The model under review builds one solid part; all positions refer to its coordinate system, in mm. A direction names the side the tool comes from. Give positions to 0.01 mm unless a question says otherwise; leave off trailing zeros. Write each loop counter-clockwise with the first axis right and the second up, starting at its lowest first coordinate (ties: lowest second). Pieces come first, ordered by that corner, then holes.
Autodesk Inventor part; units mm, degrees
ref_plane "YZ Plane" through (0, 0, 0) normal (1, 0, 0) x (0, 1, 0)
ref_plane "XZ Plane" through (0, 0, 0) normal (0, 1, 0) x (-1, 0, 0)
ref_plane "XY Plane" through (0, 0, 0) normal (0, 0, 1) x (1, 0, 0)
ref_plane "Work Plane1" through (0, 0, 0) normal (0, 0, 1) x (1, 0, 0)
sketch "Sketch1" plane through (0, 0, 0) normal (0, 0, 1) x (1, 0, 0)
  line L0 (8.0002, 76.1) -> (3.2502, 76.1) construction
  line L1 (3.2502, 90.8) -> (3.2502, 103.5) construction
  line L2 (-17.75, 107.5) -> (-17.75, -107.5) construction
  line L3 (17.75, 107.5) -> (-17.75, 107.5) construction
  line L4 (1.9802, 107.5) -> (-17.75, 107.5)
  line L5 (-17.75, 107.5) -> (-17.75, 74.83)
  line L6 (-17.75, 74.83) -> (1.9802, 74.83)
  line L7 (1.9802, 74.83) -> (1.9802, 107.5)
  line L8 (-17.75, 74.83) -> (17.75, 74.83)
  line L9 (17.75, 74.83) -> (17.75, -52.17)
  line L10 (17.75, -52.17) -> (-17.75, -52.17)
  line L11 (-17.75, -52.17) -> (-17.75, 74.83)
  point P0 (0, 0)
  dimension "d1" = 1.27
  dimension "d2" = 1.27
  dimension "d5" = 127
extrude "Extrusion1" add sketch "Sketch1" along normal blind 2.54
sketch "Sketch2" plane through (0, 0, 2.54) normal (0, 0, 1) x (1, 0, 0)
  circle A0 centre (9.0001, 13.4819) radius 34.925 construction
  line L0 (12.3751, 101.9) -> (12.3751, 92.4) construction
  line L1 (5.6252, 92.4) -> (5.6252, 101.9) construction
  line L2 (-23.5916, 26.0332) -> (5.6252, 101.9) construction
  line L3 (41.5918, 26.0331) -> (12.3751, 101.9) construction
  point P0 (0, 0)
sketch "Sketch3" plane through (0, 0, 2.54) normal (0, 0, 1) x (1, 0, 0)
  circle A0 centre (9.0001, 13.4819) radius 44.45 construction
  point P0 (0, 0)
properties part number "horizontal spool mount bottom"
1) Consider section A-A, the plane z = 2. Give the boundary of the cut face in (x, y), then the cut area to 3 significant figures.
2) Insertion check: pin 1 (0.8 mm diameter, centred on x = 11.5, z = 1, fed in from +Y); pin 2 (1.3 mm diameter, centred on y = 91, z = 1, fed in from +X). Each pin has a flat end and moves straight along its axis. Give the tip position at first contact, or say it passes through.
3) Consider section B-B, the plane x = 13.5. Give the boundary of the cut face in (y, z), then the cut area to 3 significant figures.
4) Tool access review of faces 1 (the flat face through (0, 29, 0)), 2 (the flat face through (1.98, 91, 1)): name each direction out of +Z, -Z, +X, -X, +Y, -Y from which nothing blocks a thin tool from reaching the whole face with its end or side.
5) Consider section C-C, the plane y = 83.5. Give the boundary of the cut face in (x, z), then the cut area to 3 significant figures.
6) To check wall thickness, follow probe 1 along Y at (x, z) = (7, 1.5); probe 2 along X at (y, z) = (96, 1.4). State the ranges of each line that lie inside material, in increasing order.
Answer block:
1. outline: (-17.75, -52.17) - (17.75, -52.17) - (17.75, 74.83) - (1.98, 74.83) - (1.98, 107.5) - (-17.75, 107.5) - close
1. area: 5,150 mm2
2. pin 1: stops at y = 74.83
2. pin 2: stops at x = 1.98
3. outline: (-52.17, 0) - (74.83, 0) - (74.83, 2.54) - (-52.17, 2.54) - close
3. area: 323 mm2
4. face 1: -Z, +X, -X, +Y, -Y
4. face 2: +Z, -Z, +X, +Y
5. outline: (-17.75, 0) - (1.98, 0) - (1.98, 2.54) - (-17.75, 2.54) - close
5. area: 50.1 mm2
6. probe 1: y = -52.17 to 74.83
6. probe 2: x = -17.75 to 1.98
